Can you work these out from the model? Positions are in its coordinate system, mm. Give positions to 0.01 mm unless a question says otherwise; leave off trailing zeros. Order: outer loops, then holes, each group sorted by start corner. A loop starts at its lowest first (then second) coordinate and runs counter-clockwise, first axis right, second up. Notation, with made-up numbers: M -14.5,83.5 L 22.5,83.5 A18 cw 22.5,97.5 Z; hole C 5.5,34.25 d5. An arc over 180 degrees is marked long. Answer as a JSON object with one key per item and string values.
```python
from build123d import *

# Parameters (mm, degrees)
F0_R     = 12.1285
F1_DEPTH = 6.35
F2_R     = 25.4
F3_R     = 25.4
F4_R     = 25.4


with BuildPart() as f1:
    # F0 (on Top) → F1 (new body)
    with BuildSketch(Plane.XY):
        Polygon((0, -76.487995), (65.884729, 37.627703), (-65.884729, 37.627703), align=None)
        with Locations((0, -30.727365)):
            Circle(F0_R, mode=Mode.SUBTRACT)
        with Locations((0, -0.410863)):
            Circle(F0_R, mode=Mode.SUBTRACT)
        with Locations((-26.254852, 14.747383)):
            Circle(F0_R, mode=Mode.SUBTRACT)
        with Locations((26.254857, 14.747391)):
            Circle(F0_R, mode=Mode.SUBTRACT)
    extrude(amount=F1_DEPTH)

    # F2
    f2_edges = [f1.edges().sort_by_distance(p)[0] for p in [
        (-65.884729, 37.627703, 3.175),
    ]]
    fillet(f2_edges, radius=F2_R)

    # F3
    f3_edges = [f1.edges().sort_by_distance(p)[0] for p in [
        (65.884729, 37.627703, 3.175),
    ]]
    fillet(f3_edges, radius=F3_R)

    # F4
    f4_edges = [f1.edges().sort_by_distance(p)[0] for p in [
        (0, -76.487995, 3.175),
    ]]
    fillet(f4_edges, radius=F4_R)


solid = f1.part
```
1) I want a section at A-A on x = 0. Write out the boundary of the cut face in (y, z).
Results found:
{"outline": "M -51.09,0 L -42.86,0 L -42.86,6.35 L -51.09,6.35 Z; M -18.6,0 L -12.54,0 L -12.54,6.35 L -18.6,6.35 Z; M 11.72,0 L 37.63,0 L 37.63,6.35 L 11.72,6.35 Z"}
2) I want a section at D-D on z = 4.25. Write out the boundary of the cut face in (x, y).
Results found:
{"outline": "M -43.89,-0.47 L -22,-38.39 A25.4 ccw 22,-38.39 L 43.89,-0.47 A25.4 ccw 21.89,37.63 L -21.89,37.63 A25.4 ccw Z; hole C -26.25,14.75 d24.26; hole C 0,-30.73 d24.26; hole C 0,-0.41 d24.26; hole C 26.25,14.75 d24.26"}
3) Thinking about a two-plate mould opening in Y: for faces 1 (the face through (-20.658, 3.987, 3.131)), 2 (the face through (32.789, -19.696, 3.131)), 3 (the face through (-11, -6, 0)), which applies, pulls with the +Y half, pulls with the -Y half, needs draft (parallel to the pull), parting line crosses it, or undercut?
Results found:
{"face 1": "undercut", "face 2": "pulls with the -Y half", "face 3": "needs draft"}
4) I want a section at C-C on x = 24. Write out the boundary of the cut face in (y, z), and give its area (3 significant figures).
Results found:
{"outline": "M -34.92,0 L 2.83,0 L 2.83,6.35 L -34.92,6.35 Z; M 26.66,0 L 37.54,0 L 37.54,6.35 L 26.66,6.35 Z", "area": "309 mm²"}
5) I'm going to push flat-ended pins straight in: pin 1 Ø1.5 at (x, z) = (-28.5, 1) entering from +Y; pin 2 Ø1.5 at (x, y) = (35, 21.5) entering from +Z; pin 3 Ø12 at (x, y) = (-14, 21) entering from -Z. Where does each tip first touch, or does it pass through?
Results found:
{"pin 1": "stops at y = 36.94", "pin 2": "passes through", "pin 3": "stops at z = 0"}
6) I need wall thicknesses on L1, parallel to Y at x = 0, z = 3.5; L2, parallel to Y at x = 10, z = 2.5; L3, parallel to X at y = 15.5, z = 5.75. Which ranges of each line are inside material? Lowest first, please.
Results found:
{"L1": "y = -51.09 to -42.86, -18.6 to -12.54, 11.72 to 37.63", "L2": "y = -49.04 to -37.59, -23.86 to -7.27, 6.45 to 37.63", "L3": "x = -47.08 to -38.36, -14.15 to 14.15, 38.36 to 47.08"}
7) I want a section at B-B on y = -6. Write out the boundary of the cut face in (x, z).
Results found:
{"outline": "M -40.7,0 L -10.76,0 L -10.76,6.35 L -40.7,6.35 Z; M 10.76,0 L 40.7,0 L 40.7,6.35 L 10.76,6.35 Z"}
